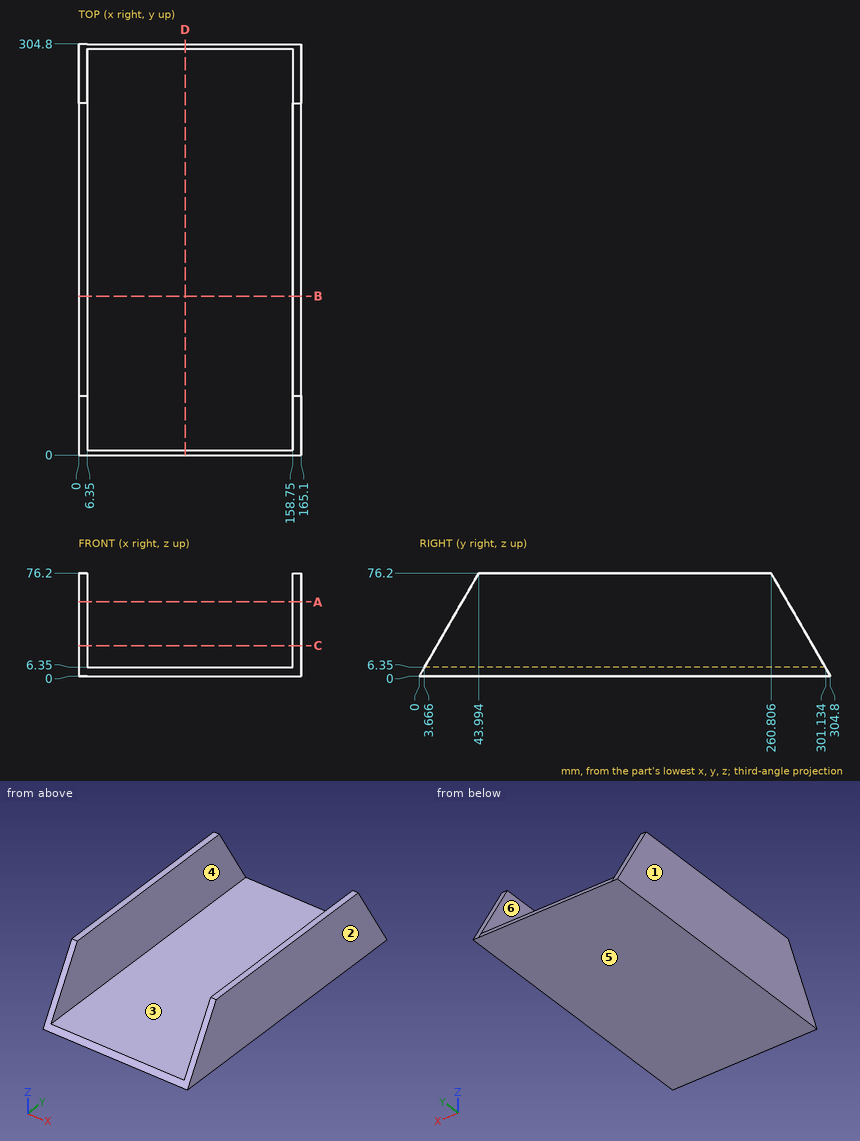
Input: dimensioned drawing with shaded views. Units: mm. Origin: part minimum x, y, z. A direction names the side the tool comes from. Coordinates: 2 decimals unless noted, no trailing zeros. Loops run counter-clockwise (first coordinate to the right, second up) from the corner with the lowest first, then second, coordinate; pieces in that order, holes last. Notation, with made-up numbers: M 46,40.5 L 87,40.5 A27 ccw 87,59.5 Z; hole C 51.25,78 d2. An arc over 180 degrees is marked long. Use a Markdown table: item, result. Add a question column.
Q1. Section query D-D, the plane x = 79. Return loops of the section in (y, z), and give its area (3 significant figures).
Q2. Draft query along X for the marked faces 1, 2, 3 and 4. Return one class per face: pulls with the +X half, pulls with the -X half, needs draft (parallel to the pull), parting line crosses it, or undercut.
Q3. Section query C-C, the plane z = 22.5. Return loops of the section in (x, y), and give its area (3 significant figures).
Q4. Access query for the marked faces 5 and 6. Directions: +Z, -Z, +X, -X, +Y, -Y. A direction counts if a zero-diameter tool reaches every point of the face in a straight line with its end or side. Return the directions, or none.
Q5. Section query B-B, the plane y = 118. Return loops of the section in (x, z).
Q6. Material intervals for L1, parallel to X at y = 101.5, z = 47.5; L2, parallel to Z at x = 73, y = 104; L3, parallel to Y at x = 35, z = 4.5, sorted ascending.
Q7. Section query A-A, the plane z = 55. Return loops of the section in (x, y).
Q8. First-contact query: pin 1 (8 mm diameter, centred on x = 25.5, z = 9.5, fed in from +Y) (1 decimal); pin 2 (8 mm diameter, centred on x = 16.5, y = 46.5, fed in from -Z); pin 3 (10 mm diameter, centred on x = 71.5, z = 10.5, fed in from -Y) (1 decimal). Flat tips, straight axial feed; report the tip coordinate or a pass-through.
Result:
| question | item | result |
|---|---|---|
| 1 | outline | M 0,0 L 304.8,0 L 301.13,6.35 L 3.67,6.35 Z |
| 1 | area | 1,910 mm2 |
| 2 | face 1 | pulls with the -X half |
| 2 | face 2 | pulls with the +X half |
| 2 | face 3 | undercut |
| 2 | face 4 | undercut |
| 3 | outline | M 0,12.99 L 6.35,12.99 L 6.35,291.81 L 0,291.81 Z; M 158.75,12.99 L 165.1,12.99 L 165.1,291.81 L 158.75,291.81 Z |
| 3 | area | 3,540 mm2 |
| 4 | face 5 | -Z, +X, -X, +Y, -Y |
| 4 | face 6 | +Z, +Y, -Y |
| 5 | outline | M 0,0 L 165.1,0 L 165.1,76.2 L 158.75,76.2 L 158.75,6.35 L 6.35,6.35 L 6.35,76.2 L 0,76.2 Z |
| 6 | L1 | x = 0 to 6.35, 158.75 to 165.1 |
| 6 | L2 | z = 0 to 6.35 |
| 6 | L3 | y = 2.6 to 302.2 |
| 7 | outline | M 0,31.75 L 6.35,31.75 L 6.35,273.05 L 0,273.05 Z; M 158.75,31.75 L 165.1,31.75 L 165.1,273.05 L 158.75,273.05 Z |
| 8 | pin 1 | stops at y = 301.6 |
| 8 | pin 2 | stops at z = 0 |
| 8 | pin 3 | stops at y = 3.2 |
